The listing builds one solid part. Answer for the finished solid, in the listing's coordinates (mm). A direction names the side the tool comes from. Give positions to 0.01 mm unless a question says otherwise; leave off trailing zeros.
```python
from build123d import *

# Parameters (mm, degrees)
BOSS_EXTRUDE1_DEPTH = 82


with BuildPart() as part:
    # Sketch4 → Boss-Extrude1 (new body, symmetric)
    with BuildSketch(Plane.XY):
        with BuildLine():
            Line((3, -10), (8.25, -10))
            ThreePointArc((8.25, -10), (9.487436867, -9.487436867), (10, -8.25))
            Line((10, -8.25), (10, -3))
            ThreePointArc((10, -3), (9.853553391, -2.646446609), (9.5, -2.5))
            Line((9.5, -2.5), (8.424621202, -2.5))
            ThreePointArc((8.424621202, -2.5), (8.071067812, -2.646446609), (7.924621202, -3))
            Line((7.924621202, -3), (7.924621202, -5.25))
            ThreePointArc((7.924621202, -5.25), (7.615962919, -5.711939766), (7.071067812, -5.603553391))
            Line((7.071067812, -5.603553391), (4.478679656, -3.011165235))
            ThreePointArc((4.478679656, -3.011165235), (3.828361402, -2.037895189), (3.6, -0.889844892))
            Line((3.6, -0.889844892), (3.6, 0))
            Line((3.6, 0), (2.15, 0))
            ThreePointArc((2.15, 0), (1.52027958, -1.52027958), (0, -2.15))
            Line((0, -2.15), (0, -3.6))
            Line((0, -3.6), (0.889844892, -3.6))
            ThreePointArc((0.889844892, -3.6), (2.037895189, -3.828361402), (3.011165235, -4.478679656))
            Line((3.011165235, -4.478679656), (5.603553391, -7.071067812))
            ThreePointArc((5.603553391, -7.071067812), (5.711939766, -7.615962919), (5.25, -7.924621202))
            Line((5.25, -7.924621202), (3, -7.924621202))
            ThreePointArc((3, -7.924621202), (2.646446609, -8.071067812), (2.5, -8.424621202))
            Line((2.5, -8.424621202), (2.5, -9.5))
            ThreePointArc((2.5, -9.5), (2.646446609, -9.853553391), (3, -10))
        make_face()
    extrude(amount=BOSS_EXTRUDE1_DEPTH, both=True)

    # Mirror1: part across plane


with BuildPart() as part_1:
    add(part.part)
    add(part.part.mirror(Plane(origin=(0, 0, 0), x_dir=(0, 0, 1), z_dir=(1, 0, 0))))

    # Mirror2: part across plane


with BuildPart() as part_2:
    add(part_1.part)
    add(part_1.part.mirror(Plane.ZX))


solid = part_2.part
```
Item 1: Which of the six approach directions +Z, -Z, +X, -X, +Y, -Y give full straight-line access (tool end or side, diameter ignored) to faces 1 (the face through (4.29, -5.76, 1.15)), 2 (the face through (-6, 10, 1))?
Conclusion:
face 1: +Z, -Z
face 2: +Z, -Z, +X, -X, +Y
Item 2: Each of these flat-tipped pins is pushed along its axis until it touches: P1, Ø0.9, axis at x = 0, z = 17.5, coming from the -Y side; P2, Ø6, axis at x = -2, z = 35.5, coming from the -Y side; P3, Ø0.5, axis at y = 0, z = -29.5, coming from the +X side; P4, Ø1.5, axis at x = 0.5, z = 3, coming from the +Y side. Where does it stop, or does it pass through?
Conclusion:
P1: stops at y = -3.6
P2: stops at y = -10
P3: stops at x = 3.6
P4: stops at y = 3.62
Item 3: Determine the mould class of faces 3 (the face through (10, -6, 1)), 4 (the face through (-4.29, 5.76, 1.15)), 5 (the face through (-10, -6, 1)), 6 (the face through (6, -10, 1)) for opening direction X: pulls with the +X half, pulls with the -X half, needs draft (parallel to the pull), parting line crosses it, or undercut.
Conclusion:
face 3: pulls with the +X half
face 4: undercut
face 5: pulls with the -X half
face 6: needs draft
Item 4: Consider probe 1 along Y at (x, z) = (-3, 72); probe 2 along Y at (x, z) = (3.5, 51.5); probe 3 along X at (y, z) = (-5.25, -5.5). Determine where each line is inside the solid, lowest interval first.
Conclusion:
probe 1: y = -10 to -7.92, -4.47 to 4.47, 7.92 to 10
probe 2: y = -10 to -7.92, -4.97 to 4.97, 7.92 to 10
probe 3: x = -10 to -7.92, -6.72 to -3.78, 3.78 to 6.72, 7.92 to 10
